from build123d import *

# Parameters (mm, degrees)
F0_R     = 10.5
F1_DEPTH = 4
F2_R     = 8
F3_DEPTH = 39
F4_W     = 7
F4_H     = 5
F6_R     = 3.5
F7_DEPTH = 2


with BuildPart() as f1:
    # F0 (on Top) → F1 (new body)
    with BuildSketch(Plane.XY):
        Circle(F0_R)
    extrude(amount=F1_DEPTH)

    # F2 (on Top) → F3 (join)
    with BuildSketch(Plane.XY):
        Circle(F2_R)
    extrude(amount=F3_DEPTH)

    # F4 (on Right) → F5 (revolve)
    with BuildSketch(Plane.YZ):
        with Locations((3.5, 41.5)):
            Rectangle(F4_W, F4_H)
    revolve(axis=Axis((0, 0, 41.5), (0, 0, -1)))

    # F6 (on face) → F7 (cut)
    with BuildSketch(Plane(origin=(0, 0, 0), x_dir=(1, 0, 0), z_dir=(0, 0, -1))):
        Circle(F6_R)
    extrude(amount=-F7_DEPTH, mode=Mode.SUBTRACT)


solid = f1.part
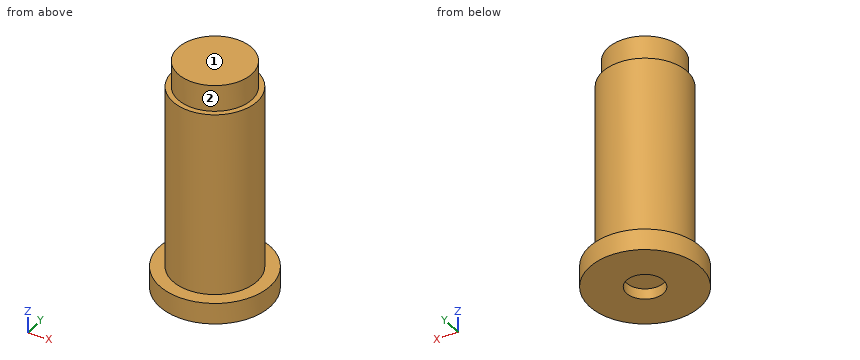
Can you work these out from the model? Positions are in its coordinate system, mm. Face numbers are marked on the shaded views. A direction names the side the tool comes from. Coordinates: 2 decimals unless noted, no trailing zeros. Write each loop counter-clockwise with the first axis right and the second up, starting at its lowest first coordinate (ties: lowest second). Pieces come first, ordered by that corner, then holes. Notation, with made-up numbers: (73, 82.25) -> (87, 82.25) arc R37 ccw to (87, 121.25) -> close; hole circle Ø1 at (69, 78.25). An arc over 180 degrees is marked (long way). Write each question's results on one line, items separated by ' | '. Start each with the question number.
Item 1: If we section it at A-A, the plane x = 0: Write out the boundary of the cut face in (y, z), and give its area (3 significant figures).
Item 2: Please list where these lines run through material, in increasing order: probe 1 along Y at (x, z) = (0, 1.25); probe 2 along Z at (x, y) = (-9.5, -4.25); probe 3 along X at (y, z) = (0, 36).
Item 3: If we section it at C-C, the plane z = 13.5: Write out the boundary of the cut face in (x, y).
Item 4: I'm going to push flat-ended pins straight in: P1, Ø2, axis at x = 0, y = -1.5, coming from the -Z side; P2, Ø10, axis at x = -1.5, y = 6, coming from the -Z side; P3, Ø3, axis at x = 0.5, z = 24, coming from the -Y side; P4, Ø10, axis at x = -1, z = 37.5, coming from the +Y side. Where does each tip first touch, or does it pass through?
Item 5: On a 3-axis mill with a long thin cutter (end or side, diameter ignored), from which of +Z, -Z, +X, -X, +Y, -Y can I reach the whole of each face in a straight line? I mean the marked faces 1 and 2. Say none if no direction works.
Item 6: If we section it at D-D, the plane y = -4.5: Write out the boundary of the cut face in (x, z), and give its area (3 significant figures).
Answer block:
1) outline: (-10.5, 0) -> (-3.5, 0) -> (-3.5, 2) -> (3.5, 2) -> (3.5, 0) -> (10.5, 0) -> (10.5, 4) -> (8, 4) -> (8, 39) -> (7, 39) -> (7, 44) -> (-7, 44) -> (-7, 39) -> (-8, 39) -> (-8, 4) -> (-10.5, 4) -> close | area: 700 mm²
2) probe 1: -10.5 to -3.5, 3.5 to 10.5 | probe 2: 0 to 4 | probe 3: -8 to 8
3) outline: circle Ø16 at (0, 0)
4) P1: z = 2 | P2: z = 0 | P3: y = -8 | P4: y = 8
5) face 1: +Z, +X, -X, +Y, -Y | face 2: +Z
6) outline: (-9.49, 0) -> (9.49, 0) -> (9.49, 4) -> (6.61, 4) -> (6.61, 39) -> (5.36, 39) -> (5.36, 44) -> (-5.36, 44) -> (-5.36, 39) -> (-6.61, 39) -> (-6.61, 4) -> (-9.49, 4) -> close | area: 593 mm²
